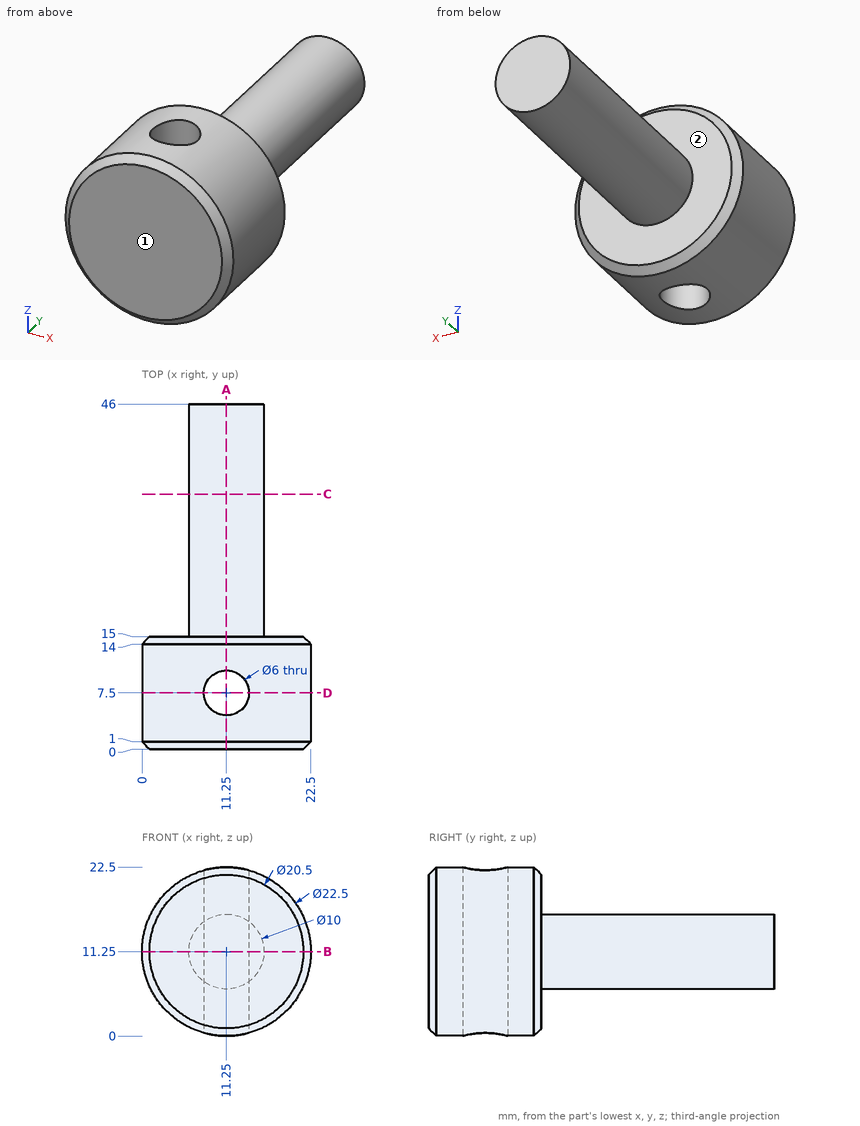
Answer from the drawing. Dimensions are ordinates in mm from the lowest x, y and z of the part. A direction names the side the tool comes from. Round coordinates to 2 decimals unless told otherwise and drop trailing zeros. Write each loop counter-clockwise with the first axis right and the second up, starting at its lowest first coordinate (ties: lowest second). Pieces come first, ordered by that corner, then holes. Notation, with made-up numbers: M 58.5,-12.75 L 65.5,-12.75 A27 cw 65.5,13.25 Z; hole C 60,4.5 d10. An arc over 180 degrees is marked long. Write each question's results on one line, items separated by ' | '. Start each with the question number.
Item 1: For the marked faces 1 and 2, determine the directions among +Z, -Z, +X, -X, +Y, -Y from which every point of the face is accessible in a straight line to the end or side of a thin tool.
Item 2: Straight lines are drawn through the part: L1, parallel to X at y = 7.5, z = 11.25; L2, parallel to Y at x = 11.25, z = 7.25; L3, parallel to Y at x = 6.75, z = 4. For each, find the intervals that lie inside material, in ascending order. Write a range as [from, to].
Item 3: A cutting plane is placed at D-D on y = 7.5. Write down the section's boundary in (x, z), and give its area (3 significant figures).
Item 4: A cutting plane is placed at B-B on z = 11.25. Write down the section's boundary in (x, y), and give its area (3 significant figures).
Item 5: A cutting plane is placed at C-C on y = 34. Write down the section's boundary in (x, z), and give its area (3 significant figures).
Item 6: A cutting plane is placed at A-A on x = 11.25. Write down the section's boundary in (y, z).
Item 7: Flat-ended cylindrical pins translate along their axes: pin 1 Ø1 at (y, z) = (16, 16) entering from +X; pin 2 Ø3 at (x, y) = (8.5, 6.5) entering from -Z; pin 3 Ø1.5 at (x, y) = (10, 17) entering from +Z. Find the tip coordinate at first contact, or state that the pin passes through.
Check sheet entries:
1) face 1: +Z, -Z, +X, -X, -Y | face 2: +Y
2) L1: [0, 8.25], [14.25, 22.5] | L2: [0, 4.5], [10.5, 46] | L3: [0, 15]
3) outline: M 8.25,0.41 L 8.25,22.09 A11.25 ccw Z; M 14.25,0.41 A11.25 ccw 14.25,22.09 Z | area: 264 mm²
4) outline: M 0,1 L 1,0 L 21.5,0 L 22.5,1 L 22.5,14 L 21.5,15 L 16.25,15 L 16.25,46 L 6.25,46 L 6.25,15 L 1,15 L 0,14 Z; hole C 11.25,7.5 d6 | area: 617 mm²
5) outline: C 11.25,11.25 d10 | area: 78.5 mm²
6) outline: M 0,1 L 1,0 L 4.5,0 L 4.5,22.5 L 1,22.5 L 0,21.5 Z; M 10.5,0 L 14,0 L 15,1 L 15,6.25 L 46,6.25 L 46,16.25 L 15,16.25 L 15,21.5 L 14,22.5 L 10.5,22.5 Z
7) pin 1: x = 13.88 | pin 2: z = 0.17 | pin 3: z = 16.22
